Can you work these out from the drawing? Everything is in mm from the part's minimum corner. Round coordinates to 2 decimals unless told otherwise and drop trailing zeros. Write each loop counter-clockwise with the first axis right and the second up, starting at its lowest first coordinate (ties: lowest second). Pieces come first, ordered by that corner, then holes. Notation, with made-up numbers: (52.5, 81.5) - (70.5, 81.5) arc R14 cw to (70.5, 100.5) - close; hole circle Ø11 at (3.5, 17). An arc over 180 degrees is marked (long way). One line per item, written item: value. Start each with the question number.
(1) Thinking about a two-plate mould opening in Y: for the marked faces 1, 2, 3 and 4, which applies, +Y half, -Y half, draft (parallel to the pull), parting line (faces both ways), or undercut?
(2) I want a section at C-C on z = 13.5. List the corners of the cut face in (x, y) for me.
(3) If I drill on L1, parallel to Y at x = 5.2, z = 3.25; L2, parallel to Y at x = 14.5, z = 15; L3, parallel to X at y = 11, z = 15.1, over which ranges is the centre line in solid material (lowest first)? Write a range as from..to.
(4) I want a section at B-B on x = 5.2. List the corners of the cut face in (y, z) for me.
(5) I want a section at D-D on x = 14.5. List the corners of the cut face in (y, z) for me, plus the area to 3 significant figures.
(6) I'm going to push a flat-ended pin straight in: pin 1 Ø3 at (x, z) = (12, 2) entering from -Y. Where does the tip first touch, or does it pass through?
(7) I want a section at A-A on y = 2.25. List the corners of the cut face in (x, z) for me.
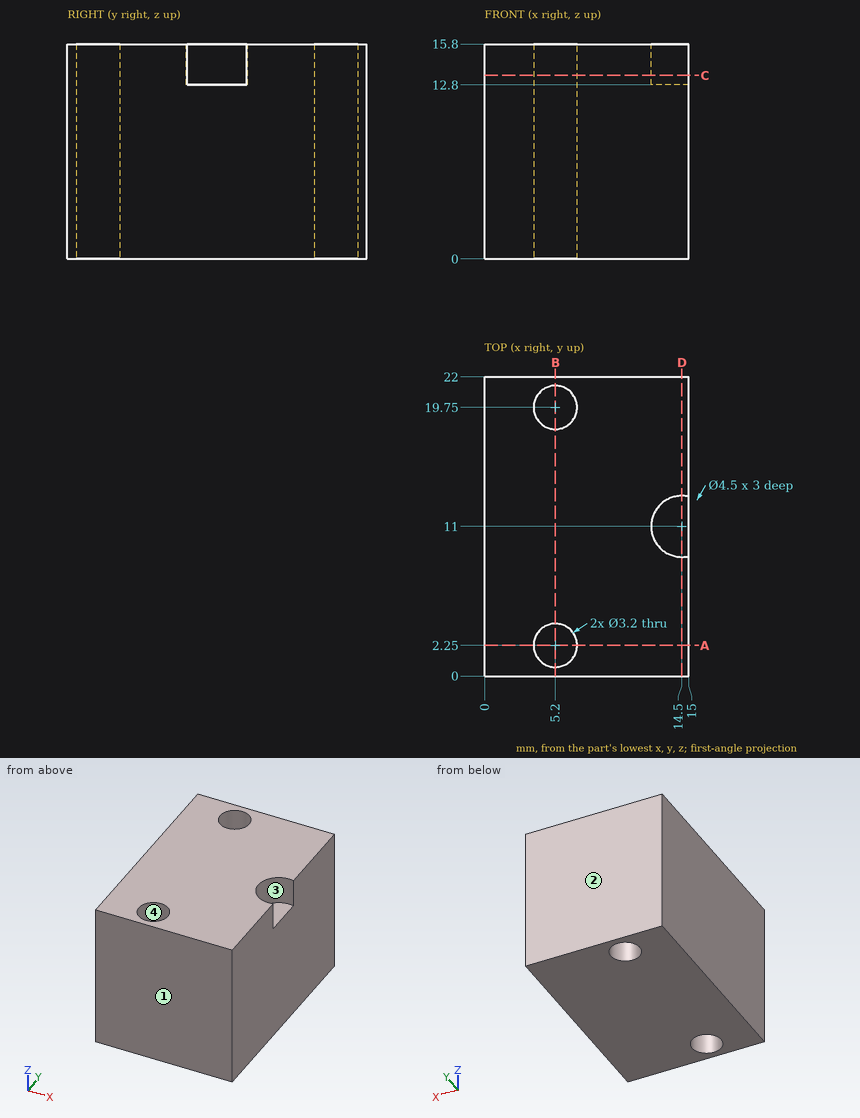
Established:
1. face 1: -Y half
1. face 2: +Y half
1. face 3: undercut
1. face 4: undercut
2. outline: (0, 0) - (15, 0) - (15, 8.81) arc R2.25 cw (long way) to (15, 13.19) - (15, 22) - (0, 22) - close; hole circle Ø3.2 at (5.2, 2.25); hole circle Ø3.2 at (5.2, 19.75)
3. L1: 0..0.65, 3.85..18.15, 21.35..22
3. L2: 0..8.75, 13.25..22
3. L3: 0..12.25
4. outline: (0, 0) - (0.65, 0) - (0.65, 15.8) - (0, 15.8) - close; (3.85, 0) - (18.15, 0) - (18.15, 15.8) - (3.85, 15.8) - close; (21.35, 0) - (22, 0) - (22, 15.8) - (21.35, 15.8) - close
5. outline: (0, 0) - (22, 0) - (22, 15.8) - (13.25, 15.8) - (13.25, 12.8) - (8.75, 12.8) - (8.75, 15.8) - (0, 15.8) - close
5. area: 334 mm2
6. pin 1: y = 0
7. outline: (0, 0) - (3.6, 0) - (3.6, 15.8) - (0, 15.8) - close; (6.8, 0) - (15, 0) - (15, 15.8) - (6.8, 15.8) - close
